Input: part model. Units: mm. Frame: model coordinates. Face numbers are marked on the shaded views. A direction names the side the tool comes from. Coordinates: 2 decimals unless noted, no trailing zeros. Loops run counter-clockwise (first coordinate to the right, second up) from the corner with the lowest first, then second, coordinate; pieces in that order, holes last.
(1) Set-up query: the marked faces 1, 2 and 3. Return all of +Z, -Z, +X, -X, +Y, -Y with unobstructed straight access to the full face (end or side cutting, diameter ignored); none if empty.
(2) Section D-D, the plane z = 1. Return loops of the section in (x, y).
(3) Section B-B, the plane y = -24. Return loops of the section in (x, z), then the cut area to 3 significant figures.
(4) Line query: L1, parallel to X at y = -60, z = -1; L2, parallel to Y at x = -10.68, z = -2.05; L3, parallel to Z at x = -10, y = -54. Output: solid intervals per line, ascending.
(5) Section C-C, the plane x = -10.68. Return loops of the section in (y, z).
(6) Contact query for flat-ended pins moving along their axis: P1, Ø22, axis at x = -5.5, y = -32, coming from the +Z side; P2, Ø3, axis at x = 10.5, z = 19.5, coming from the -Y side; P3, Ø5.5, axis at x = -10.68, y = -59.19, coming from the +Z side; P4, Ø8, axis at x = 24, z = 13, coming from the +Y side. Output: stop coordinate, or through.
(7) Section A-A, the plane z = 16. Return loops of the section in (x, y), then the cut area to 3 significant figures.
(8) Mould query, pull axis Z, two halves, no side actions, for the marked faces 4, 5, 6 and 7. Classes: released by +Z, released by -Z, zero draft, split by the parting line, or undercut.
```python
from build123d import *

# Parameters (mm, degrees)
EXTRUDE_1_DEPTH = 3
EXTRUDE_2_DEPTH = 23
EXTRUDE_3_DEPTH = 3
FILLET_1_R      = 2
EXTRUDE_START   = 4
SKETCH_4_R      = 1.7
EXTRUDE_4_DEPTH = 4
FILLET_2_R      = 3


with BuildPart() as part:
    # 草图1 → 凸台-拉伸1 (new body)
    with BuildSketch(Plane.XY):
        with BuildLine():
            Line((-16.680000946, -37.497442229), (-16.680000946, -53.997442229))
            ThreePointArc((-16.680000946, -53.997442229), (16.90757116, -40.085014335), (30.819999054, -6.497442229))
            Line((30.819999054, -6.497442229), (14.319999054, -6.497442229))
            ThreePointArc((14.319999054, -6.497442229), (5.240309271, -28.417752446), (-16.680000946, -37.497442229))
        make_face()
    extrude(amount=EXTRUDE_1_DEPTH)

    # 草图2 → 凸台-拉伸2 (add)
    with BuildSketch(Plane.XY.offset(3)):
        with BuildLine():
            Line((-16.680000946, -48.997442229), (-16.680000946, -53.997442229))
            ThreePointArc((-16.680000946, -53.997442229), (0.33591272, -50.84503159), (15.093251764, -41.806228844))
            Line((15.093251764, -41.806228844), (11.552232101, -38.265209182))
            ThreePointArc((11.552232101, -38.265209182), (-1.578346989, -46.223882389), (-16.680000946, -48.997442229))
        make_face()
        with BuildLine():
            Line((25.819999054, -6.497442229), (30.819999054, -6.497442229))
            ThreePointArc((30.819999054, -6.497442229), (27.667588415, -23.513355895), (18.628785669, -38.270694938))
            Line((18.628785669, -38.270694938), (15.087766007, -34.729675276))
            ThreePointArc((15.087766007, -34.729675276), (23.046439214, -21.599096186), (25.819999054, -6.497442229))
        make_face()
    extrude(amount=EXTRUDE_2_DEPTH)

    # 草图3 → 凸台-拉伸3 (add)
    with BuildSketch(Plane.XY.offset(26)):
        with BuildLine():
            Line((-16.680000946, -46.997442229), (-16.680000946, -53.997442229))
            ThreePointArc((-16.680000946, -53.997442229), (16.90757116, -40.085014335), (30.819999054, -6.497442229))
            Line((30.819999054, -6.497442229), (23.819999054, -6.497442229))
            ThreePointArc((23.819999054, -6.497442229), (11.957823692, -35.135266867), (-16.680000946, -46.997442229))
        make_face()
    extrude(amount=EXTRUDE_3_DEPTH)

    # 圆角1
    fillet_1_edges = [part.edges().sort_by_distance(p)[0] for p in [
        (25.819999054, -6.497442229, 14.5),
        (15.087766007, -34.729675276, 14.5),
        (11.552232101, -38.265209182, 14.5),
        (-16.680000946, -48.997442229, 14.5),
    ]]
    fillet(fillet_1_edges, radius=FILLET_1_R)

    # 草图4 → 凸台-拉伸4 (add)
    with BuildSketch(Plane(origin=(0, 0, 0), x_dir=(-1, 0, 0), z_dir=(0, 0, -1)).offset(EXTRUDE_START)):
        with BuildLine():
            Line((16.680000946, -73.672586442), (16.680000946, -37.497442229))
            ThreePointArc((16.680000946, -37.497442229), (-5.240309271, -28.417752446), (-14.319999054, -6.497442229))
            Line((-14.319999054, -6.497442229), (-50.495143267, -6.497442229))
            ThreePointArc((-50.495143267, -6.497442229), (-30.819999054, -53.997442229), (16.680000946, -73.672586442))
        make_face()
        with Locations((10.680000946, -59.187305067)):
            Circle(SKETCH_4_R, mode=Mode.SUBTRACT)
        with Locations((-36.009861892, -12.497442229)):
            Circle(SKETCH_4_R, mode=Mode.SUBTRACT)
        with BuildLine():
            Line((-41.275548631, -22.026584935), (-29.201475803, -18.791346871))
            ThreePointArc((-29.201475803, -18.791346871), (-16.90757116, -40.085014335), (4.386096304, -52.378918978))
            Line((4.386096304, -52.378918978), (1.15085824, -64.452991806))
            ThreePointArc((1.15085824, -64.452991806), (-25.746405925, -48.9238491), (-41.275548631, -22.026584935))
        make_face(mode=Mode.SUBTRACT)
    extrude(amount=-EXTRUDE_4_DEPTH)

    # 圆角2
    fillet_2_edges = [part.edges().sort_by_distance(p)[0] for p in [
        (29.201475803, -18.791346871, -2),
        (41.275548631, -22.026584935, -2),
        (-1.15085824, -64.452991806, -2),
        (-4.386096304, -52.378918978, -2),
    ]]
    fillet(fillet_2_edges, radius=FILLET_2_R)


solid = part.part
```
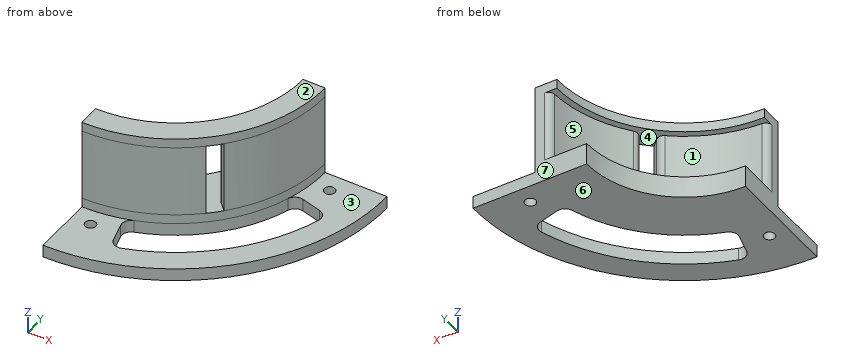
Report:
1. face 1: -X, +Y
1. face 2: +Z, +X, -X, +Y, -Y
1. face 3: +Z, +X, -Y
2. outline: (-16.68, -54) arc R47.5 ccw to (30.82, -6.5) - (14.32, -6.5) arc R31 cw to (-16.68, -37.5) - close
3. outline: (8.91, -4) - (27.48, -4) - (27.48, 29) - (19.84, 29) - (19.84, 26) - (22.05, 26) - (22.05, 3) - (8.91, 3) - close; (40.52, -4) - (48.17, -4) - (48.17, 0) - (40.52, 0) - close
3. area: 308 mm2
4. L1: x = -16.68 to -12.17, -9.19 to -2.34, 10.48 to 23.94
4. L2: y = -73.4 to -60.89, -57.49 to -36.91
4. L3: z = -4 to 0
5. outline: (-73.4, -4) - (-60.89, -4) - (-60.89, 0) - (-73.4, 0) - close; (-57.49, -4) - (-36.91, -4) - (-36.91, 3) - (-48.57, 3) - (-48.57, 26) - (-46.55, 26) - (-46.55, 29) - (-53.62, 29) - (-53.62, 0) - (-57.49, 0) - close
6. P1: stops at z = 3
6. P2: stops at y = -46.46
6. P3: stops at z = 0
6. P4: stops at y = -6.5
7. outline: (-16.68, -54) arc R47.5 ccw to (15.09, -41.81) - (12.86, -39.57) arc R2 ccw to (10.18, -39.43) arc R42.5 cw to (-14.77, -48.95) arc R2 ccw to (-16.68, -50.95) - close; (16.26, -33.36) arc R2 ccw to (16.39, -36.03) - (18.63, -38.27) arc R47.5 ccw to (30.82, -6.5) - (27.78, -6.5) arc R2 ccw to (25.78, -8.41) arc R42.5 cw to start
7. area: 325 mm2
8. face 4: undercut
8. face 5: undercut
8. face 6: released by -Z
8. face 7: zero draft
